Autodesk Inventor part; units mm, degrees
ref_plane "YZ Plane" through (0, 0, 0) normal (1, 0, 0) x (0, 1, 0)
ref_plane "XZ Plane" through (0, 0, 0) normal (0, 1, 0) x (-1, 0, 0)
ref_plane "XY Plane" through (0, 0, 0) normal (0, 0, 1) x (1, 0, 0)
sketch "Skizze1" plane through (0, 0, 0) normal (0, 1, 0) x (-1, 0, 0)
  line L0 (0, 11.18) -> (0.5, 11.18)
  line L1 (0.5, 11.18) -> (0.5, 9.98)
  line L2 (0.5, 9.98) -> (4.5, 9.98)
  line L3 (4.5, 9.98) -> (4.5, 4.515)
  line L4 (4.5, 4.515) -> (0.5, 4.515)
  line L5 (0.5, 4.515) -> (0.5, 3.515)
  line L6 (0.5, 3.515) -> (0, 3.515)
  line L7 (0, 3.515) -> (0, 11.18)
  line L8 (0, 0) -> (7.49, 0)
  dimension "d1" = 9.03
  dimension "d2" = 1
  dimension "d3" = 4
  dimension "d5" = 19.96
  dimension "d6" = 1.2
  dimension "d7" = 4
  dimension "d9" = 0.5
revolve "Umdrehung1" add sketch "Skizze1" angle 360 about axis through (0, 0, 0) along (-1, 0, 0)
sketch "Skizze2" plane through (0, 0, 0) normal (1, 0, 0) x (0, 0, -1)
  line L0 (-15.652, 0) -> (15.652, 0)
  point P0 (0, 0)
  point P1 (-8, 0)
  dimension "d11" = 8
hole "Bohrung1" at (0, 0, 8) direction (-1, 0, 0) diameter 2 depth 5 tip angle 118 countersink diameter 4 countersink angle 90
sketch "Skizze4" plane through (-4.5, 0, 0) normal (-1, 0, 0) x (0, 0, 1)
  circle A0 centre (8, 0) radius 1
  circle A1 centre (8, 0) radius 1.7
  point P0 (0, 0)
  dimension "d22" = 3.4
extrude "Extrusion1" add sketch "Skizze4" along normal blind 1.5
pattern_circular "Runde Anordnung1" count 4 over 360 about axis through (-10, 0, 0) along (1, 0, 0) of "Bohrung1", "Extrusion1"
properties part number "Getriebe Abdeckung" material "Aluminium 6061"
Could you check a few things on this model? Use its own coordinates, in mm. A direction names the side the tool comes from. Give positions to 0.01 mm unless a question says otherwise; leave off trailing zeros. Order: outer loops, then holes, each group sorted by start corner. A loop starts at its lowest first (then second) coordinate and runs counter-clockwise, first axis right, second up.
1. Suppose I cut it at B-B (z = 0). Give the number of separate pieces and of enclosed holes in the cut face, plus the area to 3 significant figures.
2. We'd pull the mould along Z, two halves only. Please class faces 3 (the cylindrical face through (-2.472, 4.408, -0.979)), 4 (the flat face through (-6, 9, 1)), 5 (the cylindrical face through (-5.24, -6.65, 1.03)), 6 (the cylindrical face through (-0.25, 3.43, -0.76)): pulls with the +Z half, pulls with the -Z half, needs draft (parallel to the pull), parting line crosses it, or undercut.
3. I need wall thicknesses on L1, parallel to Y at x = -2.6, z = 0 (3 decimals); L2, parallel to Z at x = -2.75, y = 0.5; L3, parallel to X at y = -9, z = 5.5. Which ranges of each line are inside material? Lowest first, please.
4. Suppose I cut it at C-C (y = 8). List the corners of the cut face in (x, z) for me.
5. Suppose I cut it at A-A (x = -5.2). List the corners of the cut face in (y, z) for me, plus the area to 3 significant figures.
6. Will these pins go through, and if not, where does the flat tip stop? P1, Ø1.2, axis at y = 0, z = 8, coming from the +X side; P2, Ø1, axis at x = -3, z = 2, coming from the -Y side; P3, Ø4.5, axis at y = -1, z = 1, coming from the -X side; P4, Ø2.5, axis at y = -8, z = 0, coming from the +X side.
7. For faces 1 (the flat face through (-6, 1, -9)), 2 (the cylindrical face through (-5.24, -1.03, -6.65)), which set-ups out of +Z, -Z, +X, -X, +Y, -Y let a thin tool reach every point of the face, with its end or its side?
Solved:
1. separate pieces: 4
1. enclosed holes: 0
1. area: 35.6 mm2
2. face 3: undercut
2. face 4: needs draft
2. face 5: parting line crosses it
2. face 6: undercut
3. L1: y = -9.98 to -9, -7 to -4.515, 4.515 to 7, 9 to 9.98
3. L2: z = -9.97 to -8.87, -7.13 to -4.49, 4.49 to 7.13, 8.87 to 9.97
3. L3: x = -0.5 to 0
4. outline: (-6, -1.7) - (-4.5, -1.7) - (-4.5, -5.97) - (-0.5, -5.97) - (-0.5, -7.81) - (0, -7.81) - (0, -2) - (-1, -1) - (-6, -1) - close; (-6, 1) - (-1, 1) - (0, 2) - (0, 7.81) - (-0.5, 7.81) - (-0.5, 5.97) - (-4.5, 5.97) - (-4.5, 1.7) - (-6, 1.7) - close
5. outline: circle Ø3.4 at (-8, 0); circle Ø3.4 at (0, -8); circle Ø3.4 at (0, 8); circle Ø3.4 at (8, 0); hole circle Ø2 at (-8, 0); hole circle Ø2 at (0, -8); hole circle Ø2 at (0, 8); hole circle Ø2 at (8, 0)
5. area: 23.8 mm2
6. P1: passes through
6. P2: stops at y = -9.87
6. P3: stops at x = -0.5
6. P4: stops at x = -0.75
7. face 1: +Z, -Z, -X, +Y, -Y
7. face 2: -X
